```python
from build123d import *

# Parameters (mm, degrees)
SKETCH1_W                = 500
SKETCH1_H                = 80
BOSS_EXTRUDE1_DEPTH      = 50
BOSS_EXTRUDE2_DEPTH      = 244.1
BOSS_EXTRUDE2_DEPTH_BACK = 324.1
SKETCH2_R                = 20
BOSS_EXTRUDE5_DEPTH      = 10
BOSS_EXTRUDE6_DEPTH      = 10
CUT_EXTRUDE4_DEPTH       = 613.808106347
CUT_EXTRUDE4_DEPTH_BACK  = 613.808106347
SKETCH7_R                = 20


with BuildPart() as part:
    # Sketch1 → Boss-Extrude1 (new body)
    with BuildSketch(Plane.XY):
        with Locations((91.40969163, 3.77753304)):
            Rectangle(SKETCH1_W, SKETCH1_H)
    extrude(amount=BOSS_EXTRUDE1_DEPTH)

    # Sketch2 → Boss-Extrude2 (add, two sides: drawn at the far end of the back side and taken through both)
    with BuildSketch(Plane(origin=(0, 43.77753304, 0), x_dir=(1, 0, 0), z_dir=(0, 1, 0)).offset(-BOSS_EXTRUDE2_DEPTH_BACK)):
        with Locations(Location((-158.59030837, -25, 0), (0, 0, 270))):
            Circle(SKETCH2_R)
        with Locations(Location((341.40969163, -25, 0), (0, 0, 270))):
            Circle(SKETCH2_R)
    extrude(amount=BOSS_EXTRUDE2_DEPTH + BOSS_EXTRUDE2_DEPTH_BACK)

    # Sketch5 → Boss-Extrude5 (add)
    with BuildSketch(Plane(origin=(0, -36.22246696, 0), x_dir=(-1, 0, 0), z_dir=(0, -1, 0))):
        Polygon((-341.40969163, -50), (-341.40969163, -374), (-91.40969163, -50), align=None)
    extrude(amount=-BOSS_EXTRUDE5_DEPTH)

    # Sketch6 → Boss-Extrude6 (add)
    with BuildSketch(Plane(origin=(0, 43.77753304, 0), x_dir=(1, 0, 0), z_dir=(0, 1, 0))):
        Polygon((341.40969163, -50), (91.40969163, -50), (341.40969163, -374), align=None)
    extrude(amount=-BOSS_EXTRUDE6_DEPTH)

    # Sketch7 → Cut-Extrude4 (cut, two sides: drawn at the far end of the back side and taken through both)
    with BuildSketch(Plane(origin=(0, -36.22246696, 0), x_dir=(-1, 0, 0), z_dir=(0, -1, 0)).offset(-CUT_EXTRUDE4_DEPTH_BACK)):
        with Locations(Location((-315.24921844, -299.249641509, 0), (0, 0, 90))):
            Circle(SKETCH7_R)
    extrude(amount=CUT_EXTRUDE4_DEPTH + CUT_EXTRUDE4_DEPTH_BACK, mode=Mode.SUBTRACT)


solid = part.part
```
Input: part model. Units: mm. Frame: model coordinates. A direction names the side the tool comes from. Give positions to 0.01 mm unless a question says otherwise; leave off trailing zeros. Loops run counter-clockwise (first coordinate to the right, second up) from the corner with the lowest first, then second, coordinate; pieces in that order, holes last.
1) Section query D-D on z = 25. Return the cut outline in (x, y).
A:
outline: (-178.59, -280.32) - (-138.59, -280.32) - (-138.59, -36.22) - (321.41, -36.22) - (321.41, -280.32) - (361.41, -280.32) - (361.41, 287.88) - (321.41, 287.88) - (321.41, 43.78) - (-138.59, 43.78) - (-138.59, 287.88) - (-178.59, 287.88) - close
2) Line query: L1, parallel to Y at x = 228.5, z = 151; L2, parallel to Z at x = 86.5, y = 26.5; L3, parallel to Y at x = -69, z = 48.5. Output: solid intervals per line, ascending.
A:
L1: y = -36.22 to -26.22, 33.78 to 43.78
L2: z = 0 to 50
L3: y = -36.22 to 43.78
3) Reachability of faces 4 (the cylindrical face through (361.24, -0.2, 22.4)), 5 (the flat face through (341.41, 37, 210)), 6 (the flat face through (88, 4, 50)), 7 (the flat face through (342, -280.322, 25)), 8 (the flat face through (246, -26.222, 174)) from +Z, -Z, +X, -X, +Y, -Y: full face, straight path, thin tool, end or side. Return the list, or none.
A:
face 4: none
face 5: +Z, +X, +Y, -Y
face 6: +Z, -X
face 7: +Z, -Z, +X, -X, -Y
face 8: +Z, +X, -X
4) Section query B-B on y = -130.5. Return the cut outline in (x, z), and give its area (3 significant figures).
A:
outline: circle Ø40 at (-158.59, 25); circle Ø40 at (341.41, 25)
area: 2,510 mm2
5) Contact query for flat-ended pins moving along their axis: pin 1 (2.5 mm diameter, centred on y = 9.5, z = 48.5, fed in from -X); pin 2 (1.5 mm diameter, centred on y = 19.5, z = 3.5, fed in from +X); pin 3 (1.5 mm diameter, centred on x = 125, z = 65, fed in from +Y). Output: stop coordinate, or through.
A:
pin 1: stops at x = -158.59
pin 2: stops at x = 341.41
pin 3: stops at y = 43.78
6) Section query C-C on z = 171. Return the cut outline in (x, y).
A:
outline: (184.77, -36.22) - (341.41, -36.22) - (341.41, -26.22) - (184.77, -26.22) - close; (184.77, 33.78) - (341.41, 33.78) - (341.41, 43.78) - (184.77, 43.78) - close
7) Section query A-A on z = 305. Return the cut outline in (x, y).
A:
outline: (288.17, -36.22) - (296.09, -36.22) - (296.09, -26.22) - (288.17, -26.22) - close; (288.17, 33.78) - (296.09, 33.78) - (296.09, 43.78) - (288.17, 43.78) - close; (334.4, -36.22) - (341.41, -36.22) - (341.41, -26.22) - (334.4, -26.22) - close; (334.4, 33.78) - (341.41, 33.78) - (341.41, 43.78) - (334.4, 43.78) - close
8) Mould query, pull axis X, two halves, no side actions, for faces 1 (the flat face through (270, 33.778, 138)), 2 (the cylindrical face through (295.725, -31.152, 303.585)), 3 (the flat face through (214.66, 38.85, 209.73)). Classes: released by +X, released by -X, zero draft, split by the parting line, or undercut.
A:
face 1: zero draft
face 2: undercut
face 3: released by -X
